Could you check a few things on this drawing? It's one solid part, dimensions in mm from its lowest x, y, z. Coordinates: 2 decimals unless noted, no trailing zeros. Write each loop counter-clockwise with the first axis right and the second up, starting at its lowest first coordinate (ties: lowest second). Pieces come first, ordered by that corner, then holes.
Item 1: If we mould it in two halves opening along X, with no side actions, what happens to the marked faces 1, 2 and 3? For each: pulls with the +X half, pulls with the -X half, needs draft (parallel to the pull), parting line crosses it, or undercut.
Item 2: Please list where these lines run through material, in increasing order: line 1 (X direction, y = 3.5, z = 26.5); line 2 (Z direction, x = 47.5, y = 2.25); line 3 (X direction, y = 5.5, z = 11).
Item 3: I want a section at A-A (z = 15). Please give me the cut outline in (x, y).
Item 4: I want a section at B-B (y = 4.25). Please give me the cut outline in (x, z) (3 decimals), and give its area (3 significant figures).
Item 5: I want a section at C-C (x = 64.5). Please give me the cut outline in (y, z).
Item 6: I want a section at D-D (z = 3.5). Please give me the cut outline in (x, y) (3 decimals).
Item 7: I'm going to push flat-ended pins straight in: P1, Ø5, axis at x = 29.5, z = 9.5, coming from the -Y side; P2, Ø1.5, axis at x = 20, y = 4.5, coming from the +Z side. Where does each tip first touch, or does it pass through?
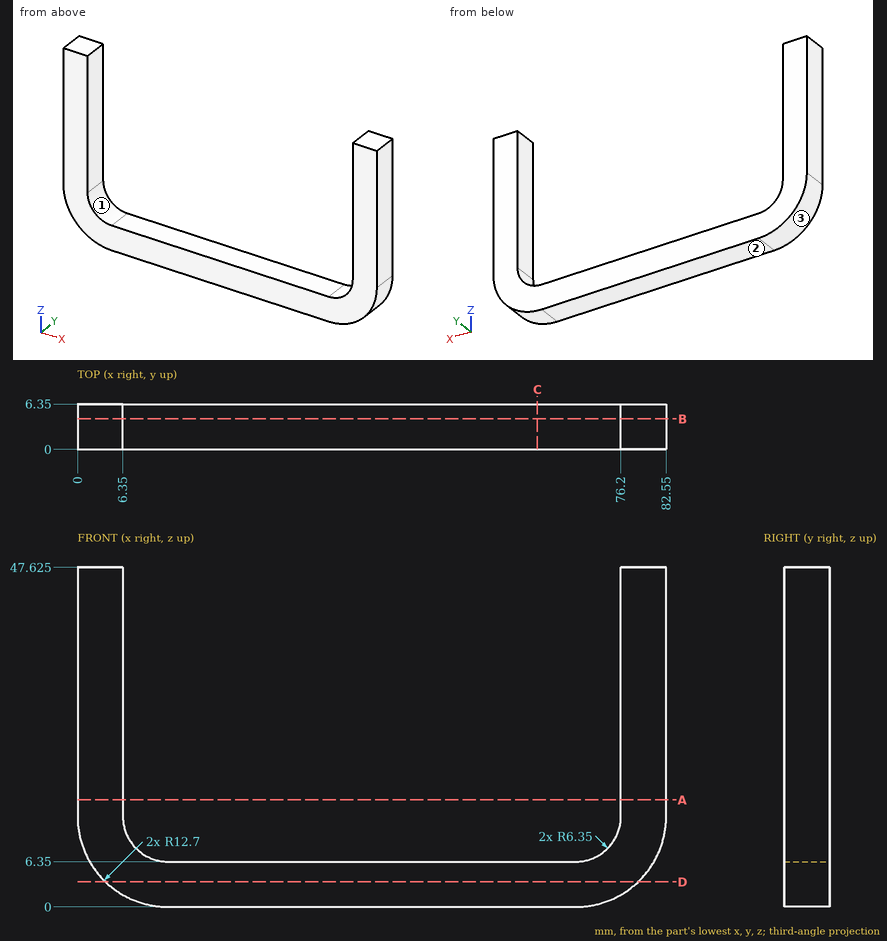
Answer:
1. face 1: undercut
1. face 2: needs draft
1. face 3: pulls with the -X half
2. line 1: x = 0 to 6.35, 76.2 to 82.55
2. line 2: z = 0 to 6.35
2. line 3: x = 0.11 to 6.58, 75.97 to 82.44
3. outline: (0, 0) - (6.35, 0) - (6.35, 6.35) - (0, 6.35) - close; (76.2, 0) - (82.55, 0) - (82.55, 6.35) - (76.2, 6.35) - close
4. outline: (0, 12.7) arc R12.7 ccw to (12.7, 0) - (69.85, 0) arc R12.7 ccw to (82.55, 12.7) - (82.55, 47.625) - (76.2, 47.625) - (76.2, 12.7) arc R6.35 cw to (69.85, 6.35) - (12.7, 6.35) arc R6.35 cw to (6.35, 12.7) - (6.35, 47.625) - (0, 47.625) - close
4. area: 996 mm2
5. outline: (0, 0) - (6.35, 0) - (6.35, 6.35) - (0, 6.35) - close
6. outline: (3.945, 0) - (78.605, 0) - (78.605, 6.35) - (3.945, 6.35) - close
7. P1: passes through
7. P2: stops at z = 6.35
